Source: CAD feature listing. Evaluate the final solid. Frame: model axes, mm. Face numbers are marked on the shaded views. A direction names the side the tool comes from. Coordinates: 2 decimals unless noted, no trailing zeros. Order: outer loops, then holes, each group sorted by start corner. A loop starts at its lowest first (then second) coordinate and runs counter-clockwise, first axis right, second up.
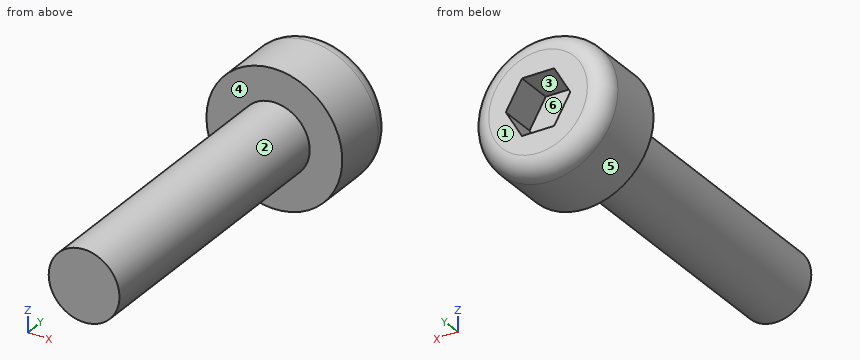
Autodesk Inventor part; units mm, degrees
ref_plane "YZ Plane" through (0, 0, 0) normal (1, 0, 0) x (0, 1, 0)
ref_plane "XZ Plane" through (0, 0, 0) normal (0, 1, 0) x (-1, 0, 0)
ref_plane "XY Plane" through (0, 0, 0) normal (0, 0, 1) x (1, 0, 0)
sketch "Sketch1" plane through (0, 0, 0) normal (0, 1, 0) x (-1, 0, 0)
  circle A0 centre (0, 0) radius 0.95
  circle A1 centre (0, 0) radius 1.825
  line L0 (0.433, -0.75) -> (-0.433, -0.75)
  line L1 (-0.433, -0.75) -> (-0.866, 0)
  line L2 (-0.866, 0) -> (-0.433, 0.75)
  line L3 (-0.433, 0.75) -> (0.433, 0.75)
  line L4 (0.433, 0.75) -> (0.866, 0)
  line L5 (0.866, 0) -> (0.433, -0.75)
  dimension "d0" = 1.9
  dimension "d1" = 3.65
  dimension "d8" = 1.5
extrude "Extrusion1" add sketch "Sketch1" along normal blind 2 contours A0 | A1 | L0 L1 L2 L3 L4 L5
extrude "Extrusion2" add sketch "Sketch1" against normal blind 8 contours A0 | L0 L1 L2 L3 L4 L5
extrude "Extrusion3" cut sketch "Sketch1" against normal blind 1 from surface at 2 contours L0 L1 L2 L3 L4 L5
fillet "Fillet1" radius 0.5 1 edges at (1.825, 2, 0)
thread "Thread2"
equation "\"d4\" = length"
equation "\"length\" = 8"
properties part number "M2x16"
1. Ray query, line 1 (Y direction, x = 1, z = 0.2); line 2 (Y direction, x = 0.4, z = 0.35); line 3 (X direction, y = -4.25, z = -0.35). Return the intervals inside material, ascending.
Findings:
line 1: y = 0 to 2
line 2: y = -8 to 1
line 3: x = -0.88 to 0.88
2. Access query for the marked faces 4, 5 and 6. Directions: +Z, -Z, +X, -X, +Y, -Y. A direction counts if a zero-diameter tool reaches every point of the face in a straight line with its end or side. Return the directions, or none.
Findings:
face 4: -Y
face 5: +Y, -Y
face 6: +Y
3. Section query A-A on x = 0. Return loops of the section in (y, z) (3 decimals).
Findings:
outline: (-8, -0.95) - (0, -0.95) - (0, -1.825) - (1.5, -1.825) arc R0.5 ccw to (2, -1.325) - (2, -0.75) - (1, -0.75) - (1, 0.75) - (2, 0.75) - (2, 1.325) arc R0.5 ccw to (1.5, 1.825) - (0, 1.825) - (0, 0.95) - (-8, 0.95) - close
4. Pin query (flat end, axial travel): P1, Ø1, axis at x = -0.5, y = -6, coming from the +Z side; P2, Ø1.5, axis at y = -0.5, z = -1.5, coming from the -X side; P3, Ø1, axis at x = 1.5, y = -1, coming from the +Z side. Return the tip coordinate at first contact, or that it passes through.
Findings:
P1: stops at z = 0.95
P2: stops at x = -1.56
P3: passes through
5. Draft query along Z for the marked faces 1, 2 and 3. Return one class per face: released by +Z, released by -Z, zero draft, split by the parting line, or undercut.
Findings:
face 1: zero draft
face 2: split by the parting line
face 3: undercut
6. Section query B-B on y = -6.5. Return loops of the section in (x, z), plus the area to 3 significant figures.
Findings:
outline: circle Ø1.9 at (0, 0)
area: 2.84 mm2
